Autodesk Inventor part; units mm, degrees
ref_plane "Work Plane1" through (0, 0, 2.5) normal (0, 0, 1) x (1, 0, 0)
ref_plane "YZ Plane" through (0, 0, 0) normal (1, 0, 0) x (0, 1, 0)
ref_plane "XZ Plane" through (0, 0, 0) normal (0, 1, 0) x (-1, 0, 0)
sketch "Sketch1" plane through (0, 0, 0) normal (0, 0, 1) x (1, 0, 0)
  line L0 (10, -10) -> (-10, -10)
  line L1 (-10, -10) -> (-10, 10)
  line L2 (-10, 10) -> (10, 10)
  line L3 (10, 10) -> (10, -10)
  line L4 (10, -10) -> (-10, 10) construction
  line L5 (-10, -10) -> (10, 10) construction
  line L6 (10, -10) -> (6, -10)
  line L7 (6, -10) -> (6, 10)
  line L8 (6, 10) -> (10, 10)
  line L9 (10, 10) -> (10, -10)
  line L10 (6, 2) -> (4, 2)
  line L11 (4, 2) -> (4, -2)
  line L12 (4, -2) -> (6, -2)
  line L13 (6, -2) -> (6, 2)
  line L14 (0, 10) -> (0, -10)
  point P0 (0, 0)
  dimension "d0" = 20
  dimension "d1" = 20
  dimension "d2" = 4
  dimension "d6" = 2
  dimension "d7" = 2
  dimension "d8" = 4
  dimension "d9" = 2
extrude "Extrusion1" add sketch "Sketch1" along normal blind 5 contours L0 L14 L2 L7 L10 L11 L12
ref_plane "Work Plane1" through (0, 0, 2.5) normal (0, 0, 1) x (1, 0, 0)
sketch "Sketch2" plane through (0, 0, 2.5) normal (0, 0, 1) x (1, 0, 0)
  line L0 (0, 10) -> (0, -10)
  line L1 (0, 3.1754) -> (2.75, 1.5877)
  line L2 (2.75, 1.5877) -> (2.75, -1.5877)
  line L3 (2.75, -1.5877) -> (0, -3.1754)
  line L4 (0, -3.1754) -> (-2.75, -1.5877)
  line L5 (-2.75, -1.5877) -> (-2.75, 1.5877)
  line L6 (-2.75, 1.5877) -> (0, 3.1754)
  point P0 (0, 0)
  point P1 (0, 0)
  dimension "d12" = 5.5
extrude "Extrusion2" cut sketch "Sketch2" along normal mid plane 1.8
sketch "Sketch3" plane through (0, 0, 5) normal (0, 0, 1) x (1, 0, 0)
  circle A0 centre (0, 0) radius 1.75
  dimension "d15" = 3.5
extrude "Extrusion3" cut sketch "Sketch3" against normal blind 8
sketch "Sketch4" plane through (0, 10, 0) normal (-1, 0, 0) x (0, 0, 1)
  circle A0 centre (2.5, -2.5) radius 1.025
  circle A1 centre (2.5, -17.5) radius 1.025
  line L0 (0, 0) -> (5, 0)
  line L1 (0, 0) -> (0, -8.25)
  line L2 (0, -11.75) -> (0, -20)
  line L3 (0, -20) -> (5, -20)
  point P0 (0, -10)
  dimension "d18" = 2.05
  dimension "d19" = 2.05
  dimension "d20" = 2.5
  dimension "d21" = 2.5
  dimension "d22" = 2.5
  dimension "d23" = 2.5
extrude "Extrusion4" cut sketch "Sketch4" against normal blind 25
sketch "Sketch5" plane through (0, 0, 0) normal (0, 0, -1) x (-1, 0, 0)
  line L0 (-6, -2) -> (-4, -2)
  line L1 (-4, -2) -> (-6, -2)
  line L2 (-6, -2) -> (-6, 2)
  line L3 (-6, 2) -> (-4, 2)
  line L4 (-4, 2) -> (-4, -2)
  point P0 (0, 0)
extrude "Extrusion5" add sketch "Sketch5" against normal blind 5
sketch "Sketch6" plane through (0, 0, 0) normal (0, 0, -1) x (-1, 0, 0)
  line L0 (-6, -10) -> (-6, 10)
  circle A0 centre (-6, 6) radius 2.5
  line L1 (-6, -9) -> (-3.5, -9)
  line L2 (-3.5, -9) -> (-3.5, -3)
  line L3 (-3.5, -3) -> (-6, -3)
  line L4 (-6, -3) -> (-6, -9)
  line L5 (0, -10) -> (-6, -10)
  line L6 (-6, 10) -> (0, 10)
  point P0 (0, 0)
  dimension "d32" = 2.5
  dimension "d33" = 1
  dimension "d34" = 6
  dimension "d35" = 5
  dimension "d36" = 4
extrude "Extrusion6" cut sketch "Sketch6" against normal blind 5
sketch "Sketch7" plane through (6, -3, 0) normal (1, 0, 0) x (0, 0, -1)
  circle A0 centre (-2.5, 3) radius 1.025
  line L0 (0, 0) -> (0, 6.5)
  line L1 (0, -7) -> (-5, -7)
  point P0 (0, 3)
  dimension "d39" = 2.5
  dimension "d40" = 10
  dimension "d41" = 2.05
extrude "Extrusion7" cut sketch "Sketch7" against normal blind 20
equation "\"d19\" = d18"
properties part number "POMSliderMotor"
Geometry check sheet. Reference: the model listing, model coordinates, mm. A direction names the side the tool comes from. Round coordinates to 2 decimals unless told otherwise and drop trailing zeros. Write each loop counter-clockwise with the first axis right and the second up, starting at its lowest first coordinate (ties: lowest second). Pieces come first, ordered by that corner, then holes. Notation, with made-up numbers: (8, 41) -> (29, 41) arc R26 cw to (29, 77) -> close; hole circle Ø2 at (-11.75, 13). An arc over 180 degrees is marked (long way). One line per item, written item: value. Start each with the question number.
(1) Scan lines: line 1 (Y direction, x = 5.75, z = 4.8); line 2 (Y direction, x = 1.1, z = 2.5) (3 decimals); line 3 (Y direction, x = 5.5, z = 0.65). Record each from-to range of solid material in increasing order. Write a range as [from, to].
(2) Cross-section at A-A, the plane y = 7.5. Record the cut outline in (x, z) (3 decimals).
(3) Cross-section at C-C, the plane z = 4.35. Record the cut outline in (x, y).
(4) Cross-section at B-B, the plane z = 2.9. Record the cut outline in (x, y).
(5) Draft check along Z on faces 4 (the flat face through (2, 0, 5)), 5 (the flat face through (1, -2, 1.6)), 6 (the flat face through (0, 6, 2)). Enter one of: +Z half, -Z half, draft (parallel to the pull), parting line (faces both ways), or undercut.
(6) Access from +Z, -Z, +X, -X, +Y, -Y to the whole of each face (thin tool, end or side, straight path). Record for faces 1 (the flat face through (3, -10, 2)), 2 (the flat face through (1, 2, 1.6)), 3 (the flat face through (5, -3, 2)).
(7) Go/stop test with flat-tipped pins: pin 1 Ø2.5 at (y, z) = (0, 2.5) entering from -X; pin 2 Ø1.5 at (y, z) = (5, 1.5) entering from +X; pin 3 Ø0.5 at (y, z) = (-1, 3) entering from -X. Record where each tip stops, or that it passes through.
(8) Cross-section at D-D, the plane y = 0. Record the cut outline in (x, z) (3 decimals), and give its area (3 significant figures).
Answer:
1. line 1: [-10, -9], [-3, 3.51], [8.49, 10]
1. line 2: [-10, -8.525], [-6.475, -2.54], [2.54, 6.475], [8.525, 10]
1. line 3: [-10, -9], [-3, 3.55], [8.45, 10]
2. outline: (0, 0) -> (4, 0) -> (4, 1.475) -> (0, 1.475) -> close; (0, 3.525) -> (4, 3.525) -> (4, 5) -> (0, 5) -> close
3. outline: (0, -10) -> (6, -10) -> (6, -9) -> (3.5, -9) -> (3.5, -3) -> (6, -3) -> (6, 3.5) arc R2.5 cw to (6, 8.5) -> (6, 10) -> (0, 10) -> (0, 1.75) arc R1.75 cw to (0, -1.75) -> close
4. outline: (0, -10) -> (6, -10) -> (6, -9) -> (3.5, -9) -> (3.5, -8.44) -> (0, -8.44) -> close; (0, -6.56) -> (3.5, -6.56) -> (3.5, -3) -> (6, -3) -> (6, -0.94) -> (2.75, -0.94) -> (2.75, -1.59) -> (0, -3.18) -> close; (0, 3.18) -> (2.75, 1.59) -> (2.75, 0.94) -> (6, 0.94) -> (6, 3.5) arc R2.5 cw to (3.56, 6.56) -> (0, 6.56) -> close; (0, 8.44) -> (5.47, 8.44) arc R2.5 cw to (6, 8.5) -> (6, 10) -> (0, 10) -> close
5. face 4: +Z half
5. face 5: undercut
5. face 6: draft
6. face 1: +Z, -Z, +X, -X, -Y
6. face 2: -X
6. face 3: +Z, -Z, +X
7. pin 1: x = 1.52
7. pin 2: x = 4.21
7. pin 3: x = 2.75
8. outline: (1.75, 0) -> (6, 0) -> (6, 1.475) -> (1.75, 1.475) -> close; (1.75, 3.525) -> (6, 3.525) -> (6, 5) -> (1.75, 5) -> close
8. area: 12.5 mm²
